from build123d import *

# Parameters (mm, degrees)
F0_W      = 457.2
F0_H      = 203.2
F1_DEPTH  = 12.7
F2_W      = 127
F2_H      = 190.5
F3_DEPTH  = 9.525
F5_D      = 11.1125
F7_DEPTH  = 3.175
F8_W      = 234.95
F8_H      = 12.7
F8_W_2    = 57.15
F8_H_2    = 285.75
F9_DEPTH  = 3.175
F10_W     = 12.7
F10_H     = 298.45
F11_DEPTH = 101.6
F13_DEPTH = 101.6
F15_D     = 14.2875
F15_DEPTH = 38.1


with BuildPart() as f1:
    # F0 (on Top) → F1 (new body)
    with BuildSketch(Plane.XY):
        Rectangle(F0_W, F0_H)
    extrude(amount=-F1_DEPTH)

    # F2 (on face) → F3 (join)
    with BuildSketch(Plane.XY):
        with Locations((158.75, 0)):
            Rectangle(F2_W, F2_H)
        with Locations((-158.75, 0)):
            Rectangle(F2_W, F2_H)
    extrude(amount=F3_DEPTH)

    # F5 (through all)
    with Locations(Plane.XY.offset(9.525)):
        with Locations((-196.85, 61.976), (-120.65, 61.976), (-196.85, -61.976), (-120.65, -61.976), (120.65, 61.976), (196.85, 61.976), (120.65, -61.976), (196.85, -61.976)):
            Hole(F5_D / 2)

    # F6 (on Front) → F7 (join, symmetric)
    with BuildSketch(Plane.XZ):
        Polygon((-87.3252, -95.25), (-87.3252, -12.7), (-214.3252, -12.7), (-214.3252, -25.4), (-100.0252, -95.25), align=None)
    extrude(amount=F7_DEPTH, both=True)

    # F8 (on Front) → F9 (join, symmetric)
    with BuildSketch(Plane.XZ):
        with Locations((99.9998, -19.05)):
            Rectangle(F8_W, F8_H)
        Polygon((-17.4752, -311.15), (217.4748, -25.4), (-17.4752, -25.4), align=None)
        with Locations((-46.0502, -19.05)):
            Rectangle(F8_W_2, F8_H)
        with Locations((-46.0502, -168.275)):
            Rectangle(F8_W_2, F8_H_2)
    extrude(amount=F9_DEPTH, both=True)

    # F10 (on Front) → F11 (join, symmetric)
    with BuildSketch(Plane.XZ):
        with Locations((-80.9752, -161.925)):
            Rectangle(F10_W, F10_H)
    extrude(amount=F11_DEPTH, both=True)

    # F12 (on Front) → F13 (join, symmetric)
    with BuildSketch(Plane.XZ):
        Polygon((-17.4752, -311.15), (-74.6252, -311.15), (-144.4752, -311.15), (-144.4752, -323.85), (-17.4752, -323.85), align=None)
    extrude(amount=F13_DEPTH, both=True)

    # F15
    with Locations(Plane(origin=(0, 0, -323.85), x_dir=(1, 0, 0), z_dir=(0, 0, -1))):
        with Locations((-125.4252, 82.55), (-125.4252, -82.55), (-36.5252, 82.55), (-36.5252, -82.55)):
            Hole(F15_D / 2, depth=F15_DEPTH)


solid = f1.part
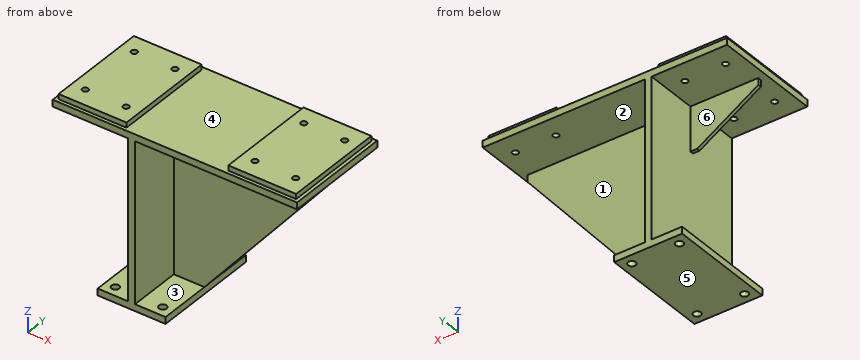
For this review, take the finished solid that the model builds, in its own axes (mm). Face numbers are marked on the shaded views. A direction names the side the tool comes from. Round coordinates to 2 decimals unless told otherwise and drop trailing zeros. Order: outer loops, then holes, each group sorted by start corner. A loop starts at its lowest first (then second) coordinate and runs counter-clockwise, first axis right, second up. Notation, with made-up numbers: (3, -16) -> (44, -16) arc R26 cw to (44, 13) -> close; hole circle Ø4 at (65.25, -35.5). An arc over 180 degrees is marked (long way). Write item = value, one per line. Start each with the question number.
1) Take a section at C-C on z = -169. State the section outline as (x, y) points (3 decimals), plus the area to 3 significant figures.
2) Take a section at A-A on y = -82.55. State the section outline as (x, z) points (3 decimals), plus the area to 3 significant figures.
3) Take a section at B-B on x = -196.85. State the section outline as (y, z) points (3 decimals), plus the area to 3 significant figures.
4) Take a section at D-D on y = -11. State the section outline as (x, z) points (3 decimals).
5) Insertion check: pin 1 (3 mm diameter, centred on x = 145.5, z = 3, fed in from -Y); pin 2 (2 mm diameter, centred on x = 99, z = -36.5, fed in from +Y) (3 decimals); pin 3 (3 mm diameter, centred on y = -79, z = -141, fed in from +X). Each pin has a flat end and moves straight along its axis. Give the tip position at first contact, or say it passes through.
6) To check wall thickness, follow line 1 (X direction, y = -82.55, z = -319.5); line 2 (Y direction, x = -196, z = 1); line 3 (Y direction, x = 120.65, z = 4.75). State the ranges of each line that lie inside material, in increasing order. Write a range as from..to.
7) The part is to be moulded in two halves that separate along Z. For the marked faces 4, 5 and 6, say which applies: +Z half, -Z half, draft (parallel to the pull), parting line (faces both ways), or undercut.
8) Tool access review of the marked faces 1, 2 and 3: name each direction out of +Z, -Z, +X, -X, +Y, -Y from which nothing blocks a thin tool from reaching the whole face with its end or side.
Verdict:
q1.outline = (-87.325, -101.6) -> (-74.625, -101.6) -> (-74.625, -3.175) -> (99.404, -3.175) -> (99.404, 3.175) -> (-74.625, 3.175) -> (-74.625, 101.6) -> (-87.325, 101.6) -> close
q1.area = 3,690 mm2
q2.outline = (-228.6, -12.7) -> (-87.325, -12.7) -> (-87.325, -311.15) -> (-118.281, -311.15) -> (-118.281, -323.85) -> (-43.669, -323.85) -> (-43.669, -311.15) -> (-74.625, -311.15) -> (-74.625, -12.7) -> (228.6, -12.7) -> (228.6, 0) -> (222.25, 0) -> (222.25, 9.525) -> (95.25, 9.525) -> (95.25, 0) -> (-95.25, 0) -> (-95.25, 9.525) -> (-222.25, 9.525) -> (-222.25, 0) -> (-228.6, 0) -> close; (-144.475, -323.85) -> (-132.569, -323.85) -> (-132.569, -311.15) -> (-144.475, -311.15) -> close; (-29.381, -323.85) -> (-17.475, -323.85) -> (-17.475, -311.15) -> (-29.381, -311.15) -> close
q2.area = 13,300 mm2
q3.outline = (-101.6, -12.7) -> (-67.532, -12.7) -> (-67.532, 9.525) -> (-95.25, 9.525) -> (-95.25, 0) -> (-101.6, 0) -> close; (-56.42, -12.7) -> (-3.175, -12.7) -> (-3.175, -36.079) -> (3.175, -36.079) -> (3.175, -12.7) -> (56.42, -12.7) -> (56.42, 9.525) -> (-56.42, 9.525) -> close; (67.532, -12.7) -> (101.6, -12.7) -> (101.6, 0) -> (95.25, 0) -> (95.25, 9.525) -> (67.532, 9.525) -> close
q3.area = 4,050 mm2
q4.outline = (-228.6, -12.7) -> (-87.325, -12.7) -> (-87.325, -311.15) -> (-144.475, -311.15) -> (-144.475, -323.85) -> (-17.475, -323.85) -> (-17.475, -311.15) -> (-74.625, -311.15) -> (-74.625, -12.7) -> (228.6, -12.7) -> (228.6, 0) -> (222.25, 0) -> (222.25, 9.525) -> (95.25, 9.525) -> (95.25, 0) -> (-95.25, 0) -> (-95.25, 9.525) -> (-222.25, 9.525) -> (-222.25, 0) -> (-228.6, 0) -> close
q5.pin_1 = -95.25
q5.pin_2 = 3.175
q5.pin_3 = -74.63
q6.line_1 = -144.48..-132.57, -118.28..-43.67, -29.38..-17.48
q6.line_2 = -95.25..-67.47, -56.49..56.49, 67.47..95.25
q6.line_3 = -95.25..-67.53, -56.42..56.42, 67.53..95.25
q7.face_4 = +Z half
q7.face_5 = -Z half
q7.face_6 = undercut
q8.face_1 = +X, +Y
q8.face_2 = +X
q8.face_3 = +X, -Y
